```python
from build123d import *

# Parameters (mm, degrees)
F1_DEPTH = 8.89


with BuildPart() as f1:
    # F0 (on Top) → F1 (new body)
    with BuildSketch(Plane.XY):
        with BuildLine():
            Line((4.445, 0), (5.715, 0))
            ThreePointArc((5.715, 0), (3.434288, 2.770181), (0, 3.81))
            Line((0, 3.81), (0, 2.54))
            ThreePointArc((0, 2.54), (2.559767, 1.860217), (4.445, 0))
        make_face()
        with BuildLine():
            Line((0, 2.54), (0, 3.81))
            ThreePointArc((0, 3.81), (-3.434288, 2.770181), (-5.715, 0))
            Line((-5.715, 0), (-4.445, 0))
            ThreePointArc((-4.445, 0), (-2.559767, 1.860217), (0, 2.54))
        make_face()
    extrude(amount=F1_DEPTH)


solid = f1.part
```
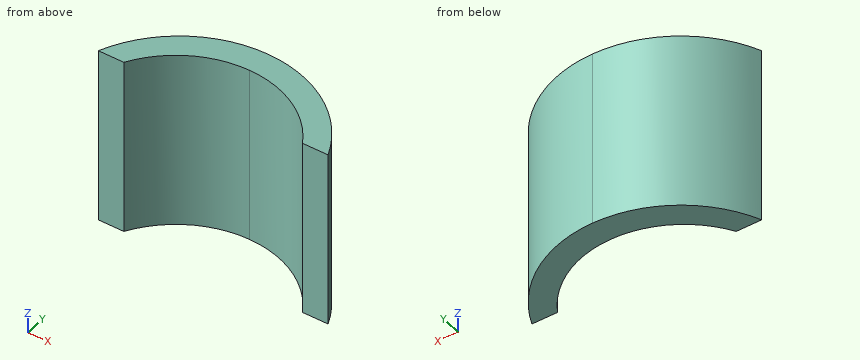
For this review, take the finished solid that the model builds, in its own axes (mm). Coordinates: 2 decimals unless noted, no trailing zeros. Loops run counter-clockwise (first coordinate to the right, second up) from the corner with the lowest first, then second, coordinate; pieces in that order, holes last.
1. Add section B-B, the plane z = 4.75. Give the boundary of the cut face in (x, y) (1 decimal), then the cut area to 3 significant figures.
2. Add section A-A, the plane y = 0.45. Give the boundary of the cut face in (x, z), then the cut area to 3 significant figures.
3. For line 1 (X direction, y = 0.3, z = 5.75); line 2 (X direction, y = 1.25, z = 6.5); line 3 (Y direction, x = -4.25, z = 8), list the stretches that pass through material, from the lowest coordinate up.
4. Add section D-D, the plane x = 3.75. Give the boundary of the cut face in (y, z).
5. Add section C-C, the plane y = 2.15. Give the boundary of the cut face in (x, z).
6. Insertion check: P1, Ø1.5, axis at x = -4, y = 0.5, coming from the +Z side; P2, Ø1.5, axis at y = 2.5, z = 3.5, coming from the -X side. Each pin has a flat end and moves straight along its axis. Give the tip position at first contact, or say it passes through.
Result:
1. outline: (-5.7, 0) - (-4.4, 0) arc R5.2 cw to (4.4, 0) - (5.7, 0) arc R6.2 ccw to start
1. area: 15.5 mm2
2. outline: (-5.51, 0) - (-4.15, 0) - (-4.15, 8.89) - (-5.51, 8.89) - close; (4.15, 0) - (5.51, 0) - (5.51, 8.89) - (4.15, 8.89) - close
2. area: 24.2 mm2
3. line 1: x = -5.58 to -4.25, 4.25 to 5.58
3. line 2: x = -5.01 to -3.41, 3.41 to 5.01
3. line 3: y = 0.31 to 2.12
4. outline: (0.92, 0) - (2.55, 0) - (2.55, 8.89) - (0.92, 8.89) - close
5. outline: (-4.22, 0) - (-1.97, 0) - (-1.97, 8.89) - (-4.22, 8.89) - close; (1.97, 0) - (4.22, 0) - (4.22, 8.89) - (1.97, 8.89) - close
6. P1: stops at z = 8.89
6. P2: stops at x = -4.61
